```python
from build123d import *

# Parameters (mm, degrees)
SKETCH_1_W          = 110
SKETCH_1_H          = 73.2
EXTRUDE_1_DEPTH     = 1
SKETCH_2_R          = 1.55
CUT_EXTRUDE_1_DEPTH = 5
FILLET_1_R          = 2
CUT_EXTRUDE_4_DEPTH = 10


with BuildPart() as part:
    # 草图1 → 凸台-拉伸1 (new body)
    with BuildSketch(Plane(origin=(0, 0, 0), x_dir=(1, 0, 0), z_dir=(0, 1, 0))):
        Rectangle(SKETCH_1_W, SKETCH_1_H)
    extrude(amount=EXTRUDE_1_DEPTH)

    # 草图2 → 切除-拉伸1 (cut)
    with BuildSketch(Plane(origin=(0, 1, 0), x_dir=(1, 0, 0), z_dir=(0, 1, 0))):
        with Locations(Location((20, 33.6, 0), (0, 0, 270))):
            Circle(SKETCH_2_R)
        with Locations(Location((40, 33.6, 0), (0, 0, 270))):
            Circle(SKETCH_2_R)
        with Locations(Location((40, -33.6, 0), (0, 0, 270))):
            Circle(SKETCH_2_R)
        with Locations(Location((20, -33.6, 0), (0, 0, 270))):
            Circle(SKETCH_2_R)
        with Locations(Location((-20, -33.6, 0), (0, 0, 270))):
            Circle(SKETCH_2_R)
        with Locations(Location((-40, -33.6, 0), (0, 0, 270))):
            Circle(SKETCH_2_R)
        with Locations(Location((-40, 33.6, 0), (0, 0, 270))):
            Circle(SKETCH_2_R)
        with Locations(Location((-20, 33.6, 0), (0, 0, 270))):
            Circle(SKETCH_2_R)
    extrude(amount=-CUT_EXTRUDE_1_DEPTH, mode=Mode.SUBTRACT)

    # 圆角1
    fillet_1_edges = [part.edges().sort_by_distance(p)[0] for p in [
        (55, 0.5, 36.6),
        (-55, 0.5, 36.6),
        (-55, 0.5, -36.6),
        (55, 0.5, -36.6),
    ]]
    fillet(fillet_1_edges, radius=FILLET_1_R)

    # 草图4 → 切除-拉伸4 (cut)
    with BuildSketch(Plane(origin=(0, 1, 0), x_dir=(1, 0, 0), z_dir=(0, 1, 0))):
        with BuildLine():
            Line((-18.384776311, 24.04163056), (24.04163056, -18.384776311))
            ThreePointArc((24.04163056, -18.384776311), (24.04163056, -24.04163056), (18.384776311, -24.04163056))
            Line((18.384776311, -24.04163056), (-24.04163056, 18.384776311))
            ThreePointArc((-24.04163056, 18.384776311), (-24.04163056, 24.04163056), (-18.384776311, 24.04163056))
        make_face()
        with BuildLine():
            Line((4.242640687, 25.455844123), (25.455844123, 4.242640687))
            ThreePointArc((25.455844123, 4.242640687), (25.455844123, -1.414213562), (19.798989873, -1.414213562))
            Line((19.798989873, -1.414213562), (-1.414213562, 19.798989873))
            ThreePointArc((-1.414213562, 19.798989873), (-1.414213562, 25.455844123), (4.242640687, 25.455844123))
        make_face()
        with BuildLine():
            Line((-25.455844123, -4.242640687), (-4.242640687, -25.455844123))
            ThreePointArc((-4.242640687, -25.455844123), (1.414213562, -25.455844123), (1.414213562, -19.798989873))
            Line((1.414213562, -19.798989873), (-19.798989873, 1.414213562))
            ThreePointArc((-19.798989873, 1.414213562), (-25.455844123, 1.414213562), (-25.455844123, -4.242640687))
        make_face()
    extrude(amount=-CUT_EXTRUDE_4_DEPTH, mode=Mode.SUBTRACT)


solid = part.part
```
Input: part model. Units: mm. Frame: model coordinates. A direction names the side the tool comes from. Coordinates: 2 decimals unless noted, no trailing zeros. Order: outer loops, then holes, each group sorted by start corner. A loop starts at its lowest first (then second) coordinate and runs counter-clockwise, first axis right, second up. Notation, with made-up numbers: (19.5, 87) - (46.5, 87) arc R33 ccw to (46.5, 119) - close; hole circle Ø9 at (14.5, 58.5). An arc over 180 degrees is marked (long way). Put each result on its own line as item: value.
1. Cut plane C-C on x = 9. Return the cut outline in (y, z), then the cut area to 3 significant figures.
Report:
outline: (0, -36.6) - (1, -36.6) - (1, -20.7) - (0, -20.7) - close; (0, -9.38) - (1, -9.38) - (1, 3.34) - (0, 3.34) - close; (0, 14.66) - (1, 14.66) - (1, 36.6) - (0, 36.6) - close
area: 50.6 mm2
2. Cut plane A-A on x = 40. Return the cut outline in (y, z).
Report:
outline: (0, -36.6) - (1, -36.6) - (1, -35.15) - (0, -35.15) - close; (0, -32.05) - (1, -32.05) - (1, 32.05) - (0, 32.05) - close; (0, 35.15) - (1, 35.15) - (1, 36.6) - (0, 36.6) - close
3. Contact query for a flat-ended pin moving along its axis: pin 1 Ø2.5 at (x, z) = (20, -33.6) entering from +Y. Output: stop coordinate, or through.
Report:
pin 1: passes through
4. Cut plane B-B on y = 0.6. State how many separate pieces and enclosed holes the cut face has, then the cut area to 3 significant figures.
Report:
separate pieces: 1
enclosed holes: 11
area: 6,880 mm2
5. Draft query along Z for faces 3 (the face through (54.4, 0.51, 36.03)), 4 (the face through (-41.375, 0.507, 34.315)), 5 (the face through (-1, 0, -9)). Return one class per face: pulls with the +Z half, pulls with the -Z half, needs draft (parallel to the pull), parting line crosses it, or undercut.
Report:
face 3: pulls with the +Z half
face 4: undercut
face 5: needs draft
6. Reachability of faces 1 (the face through (9.341, 0.507, -9.044)), 2 (the face through (-54.43, 0.51, -36)) from +Z, -Z, +X, -X, +Y, -Y: full face, straight path, thin tool, end or side. Return the list, or none.
Report:
face 1: +Y, -Y
face 2: -Z, -X, +Y, -Y
7. Line query: line 1 along X through (y, z) = (0.3, -33.6); line 2 along X through (y, z) = (0.45, 11); line 3 along X through (y, z) = (0.1, -32.5). Output: solid intervals per line, ascending.
Report:
line 1: x = -55 to -41.55, -38.45 to -21.55, -18.45 to 18.45, 21.55 to 38.45, 41.55 to 55
line 2: x = -55 to -18.7, -7.38 to 5.34, 16.66 to 55
line 3: x = -55 to -41.09, -38.91 to -21.09, -18.91 to 18.91, 21.09 to 38.91, 41.09 to 55
